Source: CAD feature listing. Evaluate the final solid. Frame: model axes, mm. Face numbers are marked on the shaded views. A direction names the side the tool comes from. Coordinates: 2 decimals unless noted, no trailing zeros. Order: outer loops, then holes, each group sorted by start corner. A loop starts at its lowest first (then second) coordinate and runs counter-clockwise, first axis right, second up.
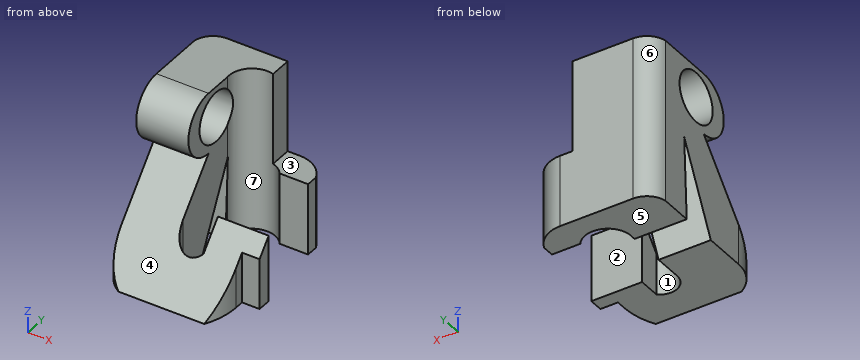
```python
from build123d import *

# Parameters (mm, degrees)
F3_DEPTH = 50
F1_R     = 15.3624630906
F4_DEPTH = 50
F5_DEPTH = 50


with BuildPart() as f3:
    # F2 (on Front) → F3 (new body, symmetric)
    with BuildSketch(Plane.XZ):
        Polygon((0, 50), (-50, 50), (-50, -50), (50, -50), (50, -6.1023989692), (0, -6.1023989692), align=None)
    extrude(amount=F3_DEPTH, both=True)

    # F1 (on Right) → F4 (intersect, symmetric)
    with BuildSketch(Plane.YZ):
        with BuildLine():
            Line((-28.1872693449, -50), (-22.0848694444, -50))
            Line((-22.0848694444, -50), (-8.4271216765, -50))
            Line((-8.4271216765, -50), (-2.9059045482, -50))
            Line((-2.9059045482, -50), (21.7942818999, 0))
            Line((21.7942818999, 0), (19.46955733, -50))
            Line((19.46955733, -50), (50, -50))
            Line((50, -50), (50, 50))
            Line((50, 50), (3.777674865, 50))
            ThreePointArc((3.777674865, 50), (-14.9746309966, 31.2476941384), (3.777674865, 12.4953882769))
            Line((3.777674865, 12.4953882769), (-50, -50))
            Line((-50, -50), (-28.1872693449, -50))
        make_face()
        with Locations((10.7518453151, 31.2476941384)):
            Circle(F1_R, mode=Mode.SUBTRACT)
    extrude(amount=F4_DEPTH, both=True, mode=Mode.INTERSECT)

    # F0 (on Top) → F5 (intersect, symmetric)
    with BuildSketch(Plane.XY):
        with BuildLine():
            Line((7.5553534552, 50), (-37.1955744922, 50))
            ThreePointArc((-37.1955744922, 50), (-45.5614657619, 46.9494015958), (-50, 39.2297059298))
            Line((-50, 39.2297059298), (-50, -28.7684518844))
            ThreePointArc((-50, -28.7684518844), (-46.7258687965, -41.0178028378), (-37.7767533064, -50))
            Line((-37.7767533064, -50), (14.8201081902, -50))
            ThreePointArc((14.8201081902, -50), (18.93844543, -39.7373000198), (20.3413292766, -28.7684518844))
            Line((20.3413292766, -28.7684518844), (20.3413292766, -23.2472326607))
            Line((20.3413292766, -23.2472326607), (31.0931764543, -23.2472326607))
            Line((31.0931764543, -23.2472326607), (31.0931764543, -14.8201109841))
            Line((31.0931764543, -14.8201109841), (0, -14.8201109841))
            Line((0, -14.8201109841), (0, -28.1872712076))
            ThreePointArc((0, -28.1872712076), (-11.6349197117, -29.9350844405), (-18.0166047066, -20.0507380068))
            Line((-18.0166047066, -20.0507380068), (-18.0166047066, 21.2131012231))
            ThreePointArc((-18.0166047066, 21.2131012231), (-9.0414378215, 36.0015865466), (7.5553534552, 31.1231197696))
            Line((7.5553534552, 31.1231197696), (24.9907784164, 31.0931745917))
            Line((24.9907784164, 31.0931745917), (24.9907784164, 38.3579358459))
            ThreePointArc((24.9907784164, 38.3579358459), (18.0378591355, 46.8219630995), (7.5553534552, 50))
        make_face()
    extrude(amount=F5_DEPTH, both=True, mode=Mode.INTERSECT)


solid = f3.part
```
1. Draft query along X for the marked faces 5, 6 and 7. Return one class per face: +X half, -X half, draft (parallel to the pull), parting line (faces both ways), or undercut.
2. Access query for the marked faces 1, 2, 3 and 4. Directions: +Z, -Z, +X, -X, +Y, -Y. A direction counts if a zero-diameter tool reaches every point of the face in a straight line with its end or side. Return the directions, or none.
3. Material intervals for line 1 along Z through (x, y) = (-42, -2); line 2 along X through (y, z) = (-18, -43.5); line 3 along Z through (x, y) = (20, 31.5), sorted ascending.
4. Section query B-B, the plane y = -1.5. Output: boundary loops of the cut face in (x, z), plus the area to 3 significant figures.
5. Section query C-C, the plane z = 34. Output: boundary loops of the cut face in (x, y).
6. Contact query for flat-ended pins moving along their axis: P1, Ø2, axis at x = 20, y = 39, coming from the +Z side; P2, Ø1.5, axis at x = -10.5, z = -23.5, coming from the -Y side; P3, Ø3, axis at x = 27.5, z = -38, coming from the -Y side. Output: stop coordinate, or through.
7. Section query D-D, the plane x = -30.5. Output: boundary loops of the cut face in (y, z).
8. Section query A-A, the plane x = 22. Output: boundary loops of the cut face in (y, z).
Answer key:
1. face 5: draft
1. face 6: -X half
1. face 7: undercut
2. face 1: +Z, -Z
2. face 2: +Z, -Z, +X
2. face 3: +Z, +X, +Y, -Y
2. face 4: +X, -X, -Y
3. line 1: z = -48.17 to 5.78, 13.41 to 22.68, 39.81 to 49.09
3. line 2: x = -50 to -18.02, 0 to 31.09
3. line 3: z = -50 to -6.1
4. outline: (-50, -47.15) - (-18.02, -47.15) - (-18.02, 6.36) - (-50, 6.36) - close; (-50, 13.25) - (-18.02, 13.25) - (-18.02, 21.98) - (-50, 21.98) - close; (-50, 40.52) - (-18.02, 40.52) - (-18.02, 49.24) - (-50, 49.24) - close
4. area: 2,270 mm2
5. outline: (-50, -14.77) - (-18.02, -14.77) - (-18.02, -4.36) - (-50, -4.36) - close; (-50, 25.87) - (-17.76, 25.87) arc R14.19 cw to (0, 36.41) - (0, 50) - (-37.2, 50) arc R13 ccw to (-50, 39.23) - close
6. P1: stops at z = -6.1
6. P2: stops at y = 34.92
6. P3: stops at y = -23.25
7. outline: (-50, -50) - (-2.91, -50) - (21.79, 0) - (19.47, -50) - (50, -50) - (50, 50) - (3.78, 50) arc R18.75 ccw to (3.78, 12.5) - close; hole circle Ø30.72 at (10.75, 31.25)
8. outline: (-23.25, -50) - (-14.82, -50) - (-14.82, -9.12) - (-23.25, -18.91) - close; (31.1, -50) - (43.28, -50) - (43.28, -6.1) - (31.1, -6.1) - close
